from build123d import *

# Parameters (mm, degrees)
F0_R     = 22.5
F0_R_2   = 20
F1_DEPTH = 3
F0_R_3   = 35
F0_R_4   = 1.6
F2_DEPTH = 3


with BuildPart() as f1:
    # F0 (on Top) → F1 (new body)
    with BuildSketch(Plane.XY):
        Circle(F0_R)
        Circle(F0_R_2, mode=Mode.SUBTRACT)
    extrude(amount=F1_DEPTH)

    # F0 (on Top) → F2 (join)
    with BuildSketch(Plane.XY):
        Circle(F0_R_3)
        with Locations((-24.681724, -14.25)):
            Circle(F0_R_4, mode=Mode.SUBTRACT)
        with Locations((0, -28.5)):
            Circle(F0_R_4, mode=Mode.SUBTRACT)
        with Locations((24.681724, -14.25)):
            Circle(F0_R_4, mode=Mode.SUBTRACT)
        with Locations((-24.681724, 14.25)):
            Circle(F0_R_4, mode=Mode.SUBTRACT)
        Circle(F0_R, mode=Mode.SUBTRACT)
        with Locations((24.681724, 14.25)):
            Circle(F0_R_4, mode=Mode.SUBTRACT)
        with Locations((0, 28.5)):
            Circle(F0_R_4, mode=Mode.SUBTRACT)
    extrude(amount=F2_DEPTH)


solid = f1.part
Geometry: final body of the model. Coordinates: model frame, mm. Coordinates: 2 decimals unless noted, no trailing zeros. Order: outer loops, then holes, each group sorted by start corner. A loop starts at its lowest first (then second) coordinate and runs counter-clockwise, first axis right, second up.
(1) Section query A-A (y = 0). Return the cut outline in (x, z).
(2) Material intervals for probe 1 along Y at (x, z) = (0, 1.7); probe 2 along X at (y, z) = (-15, 1.15); probe 3 along X at (y, z) = (-14, 2.35), sorted ascending.
(3) Section query D-D (x = 10). Return the cut outline in (y, z), plus the area to 3 significant figures.
(4) First-contact query: pin 1 (1 mm diameter, centred on y = 5, z = 1, fed in from +X); pin 2 (1.5 mm diameter, centred on y = 22, z = 0.5, fed in from +X); pin 3 (1.5 mm diameter, centred on x = 20.5, z = 2, fed in from +Y). Flat tips, straight axial feed; report the tip coordinate or a pass-through.
(5) Section query C-C (x = 0). Return the cut outline in (y, z).
(6) Section query B-B (z = 1.65). Return the cut outline in (x, y).
(7) Draft query along Y for faces 1 (the face through (15, -15, 0)), 2 (the face through (-28, -21, 1)), 3 (the face through (-0.208, -26.914, 1.479)). Return one class per face: pulls with the +Y half, pulls with the -Y half, needs draft (parallel to the pull), parting line crosses it, or undercut.
Solution:
1. outline: (-35, 0) - (-20, 0) - (-20, 3) - (-35, 3) - close; (20, 0) - (35, 0) - (35, 3) - (20, 3) - close
2. probe 1: y = -35 to -30.1, -26.9 to -20, 20 to 26.9, 30.1 to 35
2. probe 2: x = -31.62 to -26.1, -23.27 to -13.23, 13.23 to 23.27, 26.1 to 31.62
2. probe 3: x = -32.08 to -26.26, -23.1 to -14.28, 14.28 to 23.1, 26.26 to 32.08
3. outline: (-33.54, 0) - (-17.32, 0) - (-17.32, 3) - (-33.54, 3) - close; (17.32, 0) - (33.54, 0) - (33.54, 3) - (17.32, 3) - close
3. area: 97.3 mm2
4. pin 1: stops at x = 34.71
4. pin 2: stops at x = 27.81
4. pin 3: stops at y = 28.9
5. outline: (-35, 0) - (-30.1, 0) - (-30.1, 3) - (-35, 3) - close; (-26.9, 0) - (-20, 0) - (-20, 3) - (-26.9, 3) - close; (20, 0) - (26.9, 0) - (26.9, 3) - (20, 3) - close; (30.1, 0) - (35, 0) - (35, 3) - (30.1, 3) - close
6. outline: circle Ø70 at (0, 0); hole circle Ø3.2 at (-24.68, -14.25); hole circle Ø3.2 at (-24.68, 14.25); hole circle Ø40 at (0, 0); hole circle Ø3.2 at (0, -28.5); hole circle Ø3.2 at (0, 28.5); hole circle Ø3.2 at (24.68, -14.25); hole circle Ø3.2 at (24.68, 14.25)
7. face 1: needs draft
7. face 2: parting line crosses it
7. face 3: undercut
